Read the model definition and answer for the solid it produces. Units are mm, in the model's axes. Face numbers are marked on the shaded views. A direction names the side the tool comes from. Round coordinates to 2 decimals unless told otherwise and drop trailing zeros. Loops run counter-clockwise (first coordinate to the right, second up) from the corner with the lowest first, then second, coordinate; pieces in that order, holes last. Notation, with made-up numbers: M 77.25,22.5 L 103.25,22.5 A21 cw 103.25,52.5 Z; hole C -3.75,-18.75 d5. An arc over 180 degrees is marked long. Write each question's results on one line, items separated by ' | '.
from build123d import *

# Parameters (mm, degrees)
F1_DEPTH = 20
F3_DEPTH = 260
F5_DEPTH = 400


with BuildPart() as f1:
    # F0 (on Front) → F1 (new body)
    with BuildSketch(Plane.XZ):
        Polygon((-4521.589086, -1323.485495), (-5001.589086, -1323.485495), (-5001.589086, -1503.808054), (-4521.589086, -1623.485495), align=None)
    extrude(amount=F1_DEPTH)

    # F2 (on face) → F3 (join)
    with BuildSketch(Plane.XZ.offset(20)):
        Polygon((-4521.589086, -1323.485495), (-5001.589086, -1323.485495), (-5001.589086, -1503.808054), (-4981.589086, -1508.794614), (-4981.589086, -1343.485495), (-4541.589086, -1343.485495), (-4541.589086, -1618.498935), (-4521.589086, -1623.485495), align=None)
    extrude(amount=F3_DEPTH)

    # F4 (on face) → F5 (join)
    with BuildSketch(Plane(origin=(0, 0, 0), x_dir=(-1, 0, 0), z_dir=(0, 1, 0))):
        Polygon((5006.427524, -1523.213969), (5001.589086, -1503.808054), (4521.589086, -1623.485495), (4526.427524, -1642.89141), align=None)
    extrude(amount=-F5_DEPTH)


solid = f1.part
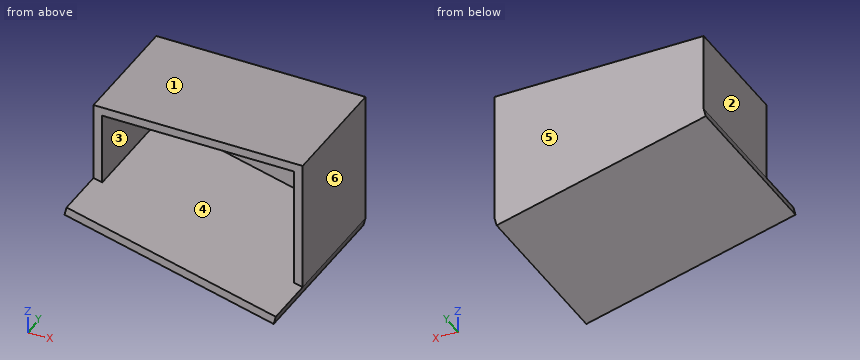
Item 1: The part is cut by section B-B (z = -1360). Determine the outline of the cut face in (x, y), plus the area to 3 significant figures.
Outcome:
outline: M -5001.59,-280 L -4981.59,-280 L -4981.59,-20 L -4541.59,-20 L -4541.59,-280 L -4521.59,-280 L -4521.59,0 L -5001.59,0 Z | area: 20,000 mm2
Item 2: The part is cut by section C-C (x = -4793). Determine the outline of the cut face in (y, z), plus the area to 3 significant figures.
Outcome:
outline: M -400,-1576.43 L 0,-1576.43 L 0,-1323.49 L -280,-1323.49 L -280,-1343.49 L -20,-1343.49 L -20,-1555.82 L -400,-1555.82 Z | area: 18,100 mm2
Item 3: For the marked faces 1, 2 and 3, determine the directions among +Z, -Z, +X, -X, +Y, -Y from which every point of the face is accessible in a straight line to the end or side of a thin tool.
Outcome:
face 1: +Z, +X, -X, +Y, -Y | face 2: +Z, -X, +Y, -Y | face 3: -Y
Item 4: Straight lines are drawn through the part: line 1 (X direction, y = -48.5, z = -1457); line 2 (Z direction, x = -4951.5, y = -212); line 3 (Z direction, x = -4617.5, y = -98). For each, find the intervals that lie inside material, in ascending order.
Outcome:
line 1: x = -5001.59 to -4981.59, -4541.59 to -4521.59 | line 2: z = -1536.91 to -1516.3, -1343.49 to -1323.49 | line 3: z = -1620.18 to -1599.57, -1343.49 to -1323.49
Item 5: The mould has two halves that part along X. Classify the marked faces 4, 5 and 6: pulls with the +X half, pulls with the -X half, needs draft (parallel to the pull), parting line crosses it, or undercut.
Outcome:
face 4: undercut | face 5: needs draft | face 6: pulls with the +X half
Item 6: The part is cut by section A-A (y = -67.5). Determine the outline of the cut face in (x, z), plus the area to 3 significant figures.
Outcome:
outline: M -5006.43,-1523.21 L -4526.43,-1642.89 L -4521.59,-1623.49 L -4521.59,-1323.49 L -5001.59,-1323.49 L -5001.59,-1503.81 Z; hole M -4981.59,-1508.79 L -4541.59,-1618.5 L -4541.59,-1343.49 L -4981.59,-1343.49 Z | area: 28,300 mm2
Item 7: Flat-ended cylindrical pins translate along their axes: pin 1 (3 mm diameter, centred on x = -4785.5, z = -1546.5, fed in from -Y); pin 2 (4 mm diameter, centred on x = -4942, y = -290, fed in from -Z); pin 3 (10 mm diameter, centred on x = -4821.5, y = -340.5, fed in from -Z). Find the tip coordinate at first contact, or state that the pin passes through.
Outcome:
pin 1: stops at y = -20 | pin 2: stops at z = -1539.78 | pin 3: stops at z = -1570.57
Item 8: The part is cut by section D-D (y = -305). Determine the outline of the cut face in (x, z), plus the area to 3 significant figures.
Outcome:
outline: M -5006.43,-1523.21 L -4526.43,-1642.89 L -4521.59,-1623.49 L -5001.59,-1503.81 Z | area: 9,890 mm2
